Build history of the part. All positions in model axes, mm. Face numbers are marked on the shaded views. Give positions to 0.01 mm unless a question says otherwise; leave off trailing zeros. Write each loop counter-clockwise with the first axis right and the second up, starting at its lowest first coordinate (ties: lowest second). Pieces come first, ordered by that corner, then holes.
from build123d import *

# Parameters (mm, degrees)
SKETCH1_R           = 38.1
BOSS_EXTRUDE1_DEPTH = 241.3
SKETCH3_R           = 330.2
SKETCH3_R_2         = 19.05
SKETCH3_R_3         = 25.4
SKETCH3_R_4         = 15.875
CUT_EXTRUDE1_DEPTH  = 228.6


with BuildPart() as part:
    # Sketch1 → Boss-Extrude1 (new, symmetric)
    with BuildSketch(Plane.XY):
        with BuildLine():
            Line((-152.4, 63.5), (-42.121134838, 63.5))
            ThreePointArc((-42.121134838, 63.5), (0, 76.2), (42.121134838, 63.5))
            Line((42.121134838, 63.5), (266.7, 63.5))
            ThreePointArc((266.7, 63.5), (330.2, 0), (266.7, -63.5))
            Line((266.7, -63.5), (42.121134838, -63.5))
            ThreePointArc((42.121134838, -63.5), (0, -76.2), (-42.121134838, -63.5))
            Line((-42.121134838, -63.5), (-152.4, -63.5))
            ThreePointArc((-152.4, -63.5), (-215.9, 0), (-152.4, 63.5))
        make_face()
        with Locations(Location((0, 0, 0), (0, 0, 180))):
            Circle(SKETCH1_R, mode=Mode.SUBTRACT)
    extrude(amount=BOSS_EXTRUDE1_DEPTH, both=True)

    # Sketch3 → Cut-Extrude1 (cut, symmetric)
    # profile 1 of 2: a face of its own
    with BuildSketch(Plane.XY):
        Circle(SKETCH3_R)
        with Locations((-152.4, 0)):
            Circle(SKETCH3_R_2, mode=Mode.SUBTRACT)
        with Locations((266.7, 0)):
            Circle(SKETCH3_R_3, mode=Mode.SUBTRACT)
    # profile 2 of 2: a face of its own
    with BuildSketch(Plane.XY):
        with Locations((-152.4, 0)):
            Circle(SKETCH3_R_4)
    extrude(amount=CUT_EXTRUDE1_DEPTH, both=True, mode=Mode.SUBTRACT)


solid = part.part
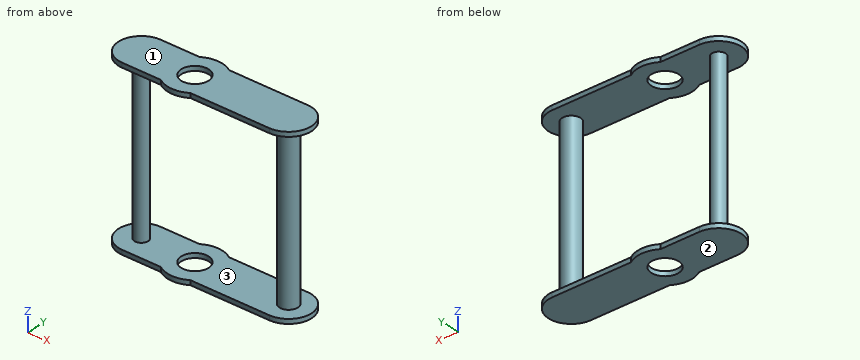
(1) Drop flat-ended pins along their axis: pin 1 (6 mm diameter, centred on y = 23.5, z = -187.5, fed in from -X); pin 2 (6.5 mm diameter, centred on x = 200, z = 237.5, fed in from -Y); pin 3 (4 mm diameter, centred on y = -20, z = 51, fed in from +X). Give the stop position or say it passes through.
(2) Saw through at D-D, the plane z = -177. List the corners of the cut face in (x, y) (3 decimals).
(3) Saw through at A-A, the plane y = 0. List the corners of the cut face in (x, z) (3 decimals), plus the area to 3 significant figures.
(4) Saw through at C-C, the plane x = 68.5. List the corners of the cut face in (y, z), plus the area to 3 significant figures.
(5) Mould opens along Z. For the marked faces 1, 2 and 3 say: +Z half, -Z half, draft (parallel to the pull), parting line (faces both ways), or undercut.
(6) Probe line 1 (Z direction, x = 238.5, y = 30.5); line 2 (Y direction, x = -152.4, z = -52.5) (3 decimals); line 3 (X direction, y = 2.5, z = 220). List the from-to ranges inside material, lowest first.
(7) Saw through at B-B, the plane x = 0. List the corners of the cut face in (y, z), plus the area to 3 significant figures.
Computed values:
1. pin 1: stops at x = 251.7
1. pin 2: stops at y = -63.5
1. pin 3: stops at x = 284.62
2. outline: circle Ø38.1 at (-152.4, 0); circle Ø50.8 at (266.7, 0); hole circle Ø31.75 at (-152.4, 0)
3. outline: (-215.9, -241.3) - (-38.1, -241.3) - (-38.1, -228.6) - (-133.35, -228.6) - (-133.35, 228.6) - (-38.1, 228.6) - (-38.1, 241.3) - (-215.9, 241.3) - (-215.9, 228.6) - (-171.45, 228.6) - (-171.45, -228.6) - (-215.9, -228.6) - close; (38.1, -241.3) - (330.2, -241.3) - (330.2, -228.6) - (292.1, -228.6) - (292.1, 228.6) - (330.2, 228.6) - (330.2, 241.3) - (38.1, 241.3) - (38.1, 228.6) - (241.3, 228.6) - (241.3, -228.6) - (38.1, -228.6) - close; hole (-168.275, -228.6) - (-136.525, -228.6) - (-136.525, 228.6) - (-168.275, 228.6) - close
3. area: 38,100 mm2
4. outline: (-63.5, -241.3) - (63.5, -241.3) - (63.5, -228.6) - (-63.5, -228.6) - close; (-63.5, 228.6) - (63.5, 228.6) - (63.5, 241.3) - (-63.5, 241.3) - close
4. area: 3,230 mm2
5. face 1: +Z half
5. face 2: -Z half
5. face 3: undercut
6. line 1: z = -241.3 to -228.6, 228.6 to 241.3
6. line 2: y = -19.05 to -15.875, 15.875 to 19.05
6. line 3: x = -171.29 to -168.08, -136.72 to -133.51, 241.42 to 291.98
7. outline: (-76.2, -241.3) - (-38.1, -241.3) - (-38.1, -228.6) - (-76.2, -228.6) - close; (-76.2, 228.6) - (-38.1, 228.6) - (-38.1, 241.3) - (-76.2, 241.3) - close; (38.1, -241.3) - (76.2, -241.3) - (76.2, -228.6) - (38.1, -228.6) - close; (38.1, 228.6) - (76.2, 228.6) - (76.2, 241.3) - (38.1, 241.3) - close
7. area: 1,940 mm2
